Design review of the part built by this model. Coordinates are the model's own, in mm. Coordinates: 2 decimals unless noted, no trailing zeros. Order: outer loops, then holes, each group sorted by start corner. A loop starts at its lowest first (then second) coordinate and runs counter-clockwise, first axis right, second up. Notation, with made-up numbers: (85, 25.5) -> (95, 25.5) arc R14 ccw to (95, 30.5) -> close; hole circle Ø3 at (30, -4.5). An arc over 180 degrees is marked (long way). Use a Markdown table: item, result. Add a question column.
Q1. Add section C-C (y = -3.3). Count the separate pieces of the cut face and the enclosed holes in it, then the cut area to 3 significant figures.
Q2. Wall thickness on probe 1 along Z at (x, y) = (30, -1.85); probe 2 along X at (y, z) = (-2.5, -9.5); probe 3 along X at (y, z) = (-0.4, 12): over which ranges is each line inside the solid? List them lowest first.
Q3. Add section D-D (x = 30). State the section outline as (y, z) points, then the cut area to 3 significant figures.
Q4. Insertion check: pin 1 (1.5 mm diameter, centred on x = 58.5, z = -11.5, fed in from +Y); pin 2 (1.5 mm diameter, centred on y = -1.5, z = -31.5, fed in from +X). Each pin has a flat end and moves straight along its axis. Give the tip position at first contact, or say it passes through.
Q5. Add section B-B (x = 90). State the section outline as (y, z) points, then the cut area to 3 significant figures.
Q6. Add section A-A (z = 10). State the section outline as (x, y) points, then the cut area to 3 significant figures.
Q7. The part is to be moulded in two halves that separate along X. For faces 1 (the face through (9.46, -1.97, -42.44)), 2 (the face through (99.27, -1.97, 19.51)), 3 (the face through (9.46, -1.97, 37.56)), 4 (the face through (38, -4, 1)), say which applies: pulls with the +X half, pulls with the -X half, needs draft (parallel to the pull), parting line crosses it, or undercut.
from build123d import *

# Parameters (mm, degrees)
F0_R     = 2.5
F1_DEPTH = 4


with BuildPart() as f1:
    # F0 (on Front) → F1 (new body)
    with BuildSketch(Plane.XZ):
        with BuildLine():
            Line((0, 48), (0, 0))
            Line((0, 0), (0, -48))
            ThreePointArc((0, -48), (0.585786, -49.414214), (2, -50))
            Line((2, -50), (38.81966, -50))
            ThreePointArc((38.81966, -50), (39.968425, -49.866245), (41.055728, -49.472136))
            Line((41.055728, -49.472136), (97.236068, -21.381966))
            ThreePointArc((97.236068, -21.381966), (99.253254, -19.538486), (100, -16.90983))
            Line((100, -16.90983), (100, 0))
            Line((100, 0), (100, 16.90983))
            ThreePointArc((100, 16.90983), (99.253254, 19.538486), (97.236068, 21.381966))
            Line((97.236068, 21.381966), (41.055728, 49.472136))
            ThreePointArc((41.055728, 49.472136), (39.968425, 49.866245), (38.81966, 50))
            Line((38.81966, 50), (2, 50))
            ThreePointArc((2, 50), (0.585786, 49.414214), (0, 48))
        make_face()
        with Locations((10, -40)):
            Circle(F0_R, mode=Mode.SUBTRACT)
        with Locations((30, -40)):
            Circle(F0_R, mode=Mode.SUBTRACT)
        with Locations((50, -10)):
            Circle(F0_R, mode=Mode.SUBTRACT)
        with Locations((90, -10)):
            Circle(F0_R, mode=Mode.SUBTRACT)
        with Locations((10, 0)):
            Circle(F0_R, mode=Mode.SUBTRACT)
        with Locations((30, 0)):
            Circle(F0_R, mode=Mode.SUBTRACT)
        with Locations((10, 40)):
            Circle(F0_R, mode=Mode.SUBTRACT)
        with Locations((30, 40)):
            Circle(F0_R, mode=Mode.SUBTRACT)
        with Locations((50, 10)):
            Circle(F0_R, mode=Mode.SUBTRACT)
        with Locations((90, 10)):
            Circle(F0_R, mode=Mode.SUBTRACT)
    extrude(amount=F1_DEPTH)


solid = f1.part
Established:
| question | item | result |
|---|---|---|
| 1 | separate pieces | 1 |
| 1 | enclosed holes | 10 |
| 1 | area | 8,000 mm^2 |
| 2 | probe 1 | -50 to -42.5, -37.5 to -2.5, 2.5 to 37.5, 42.5 to 50 |
| 2 | probe 2 | 0 to 47.55, 52.45 to 87.55, 92.45 to 100 |
| 2 | probe 3 | 0 to 48.5, 51.5 to 88.5, 91.5 to 100 |
| 3 | outline | (-4, -50) -> (0, -50) -> (0, -42.5) -> (-4, -42.5) -> close; (-4, -37.5) -> (0, -37.5) -> (0, -2.5) -> (-4, -2.5) -> close; (-4, 2.5) -> (0, 2.5) -> (0, 37.5) -> (-4, 37.5) -> close; (-4, 42.5) -> (0, 42.5) -> (0, 50) -> (-4, 50) -> close |
| 3 | area | 340 mm^2 |
| 4 | pin 1 | y = 0 |
| 4 | pin 2 | x = 78.5 |
| 5 | outline | (-4, -25) -> (0, -25) -> (0, -12.5) -> (-4, -12.5) -> close; (-4, -7.5) -> (0, -7.5) -> (0, 7.5) -> (-4, 7.5) -> close; (-4, 12.5) -> (0, 12.5) -> (0, 25) -> (-4, 25) -> close |
| 5 | area | 160 mm^2 |
| 6 | outline | (0, -4) -> (47.5, -4) -> (47.5, 0) -> (0, 0) -> close; (52.5, -4) -> (87.5, -4) -> (87.5, 0) -> (52.5, 0) -> close; (92.5, -4) -> (100, -4) -> (100, 0) -> (92.5, 0) -> close |
| 6 | area | 360 mm^2 |
| 7 | face 1 | undercut |
| 7 | face 2 | pulls with the +X half |
| 7 | face 3 | undercut |
| 7 | face 4 | needs draft |
